Autodesk Inventor part; units mm, degrees
ref_plane "Work Plane5" through (-4.7625, 0, 3.175) normal (0, 0, 1) x (1, 0, 0)
ref_plane "YZ Plane" through (0, 0, 0) normal (1, 0, 0) x (0, 1, 0)
ref_plane "XZ Plane" through (0, 0, 0) normal (0, 1, 0) x (-1, 0, 0)
sketch "Sketch1" plane through (0, 0, 0) normal (0, 1, 0) x (-1, 0, 0)
  line L0 (-6.35, 12.7) -> (6.35, 12.7)
  line L1 (6.35, 12.7) -> (6.35, -12.7)
  line L2 (6.35, -12.7) -> (-6.35, -12.7)
  line L3 (-6.35, -12.7) -> (-6.35, 12.7)
  line L4 (-6.35, 12.7) -> (6.35, -12.7) construction
  line L5 (6.35, 12.7) -> (-6.35, -12.7) construction
  line L6 (-9.525, 19.05) -> (9.525, 19.05)
  line L7 (9.525, 19.05) -> (9.525, -19.05)
  line L8 (9.525, -19.05) -> (-9.525, -19.05)
  line L9 (-9.525, -19.05) -> (-9.525, 19.05)
  line L10 (-9.525, 19.05) -> (9.525, -19.05) construction
  line L11 (9.525, 19.05) -> (-9.525, -19.05) construction
  line L12 (6.35, 12.7) -> (6.35, 15.875)
  line L13 (6.35, 15.875) -> (9.525, 15.875)
  point P0 (0, 0)
  dimension "d0" = 12.7
  dimension "d1" = 25.4
extrude "Extrusion1" add sketch "Sketch1" along normal blind 3.175
sketch "Sketch2" plane through (0, 3.175, 0) normal (0, 1, 0) x (1, 0, 0)
  circle A0 centre (3.175, -9.525) radius 1.5875
  circle A1 centre (-3.175, 0) radius 1.5875
  circle A2 centre (0, 8.5298) radius 1.5
  line L0 (-4.318, -7.9375) -> (-2.032, -7.9375)
  line L1 (-2.032, -7.9375) -> (-2.032, -11.1125)
  line L2 (-2.032, -11.1125) -> (-4.318, -11.1125)
  line L3 (-4.318, -11.1125) -> (-4.318, -7.9375)
  line L4 (-4.318, -7.9375) -> (-2.032, -11.1125) construction
  line L5 (-2.032, -7.9375) -> (-4.318, -11.1125) construction
  line L6 (-9.525, 19.05) -> (-9.525, -19.05)
  line L7 (9.525, -19.05) -> (-9.525, -19.05)
  line L8 (-9.525, -19.05) -> (-9.525, 19.05)
  line L9 (-9.525, 19.05) -> (9.525, 19.05)
  line L10 (9.525, 19.05) -> (9.525, -19.05)
  line L11 (9.525, -19.05) -> (-9.525, 19.05) construction
  line L12 (-9.525, -19.05) -> (9.525, 19.05) construction
  point P0 (0, 0)
  point P1 (0, 0)
  dimension "d4" = 3.175
  dimension "d5" = 3.175
  dimension "d6" = 3
  dimension "d8" = 3.175
extrude "Extrusion2" add sketch "Sketch2" along normal blind 3.175
sketch "Sketch3" plane through (0, 6.35, 0) normal (0, 1, 0) x (1, 0, 0)
  line L0 (-9.525, 19.05) -> (-9.525, -19.05)
  line L1 (9.525, -19.05) -> (-9.525, -19.05)
  line L2 (-9.525, -19.05) -> (-9.525, 19.05)
  line L3 (-9.525, 19.05) -> (9.525, 19.05)
  line L4 (9.525, 19.05) -> (9.525, -19.05)
  line L5 (9.525, -19.05) -> (-9.525, 19.05) construction
  line L6 (-9.525, -19.05) -> (9.525, 19.05) construction
  line L7 (6.35, -12.7) -> (-6.35, -12.7)
  line L8 (-6.35, -12.7) -> (-6.35, 12.7)
  line L9 (-6.35, 12.7) -> (6.35, 12.7)
  line L10 (6.35, 12.7) -> (6.35, -12.7)
  line L11 (6.35, -12.7) -> (-6.35, 12.7) construction
  line L12 (-6.35, -12.7) -> (6.35, 12.7) construction
  point P0 (0, 0)
extrude "Extrusion3" add sketch "Sketch3" along normal blind 3.175
sketch "Sketch4" plane through (9.525, 0, -19.05) normal (0, 0, -1) x (-1, 0, 0)
  line L0 (12.7, 0) -> (6.35, 0)
  line L1 (6.35, 0) -> (6.35, 9.525)
  line L2 (6.35, 9.525) -> (12.7, 9.525)
  line L3 (12.7, 9.525) -> (12.7, 0)
  line L4 (12.7, 0) -> (6.35, 9.525) construction
  line L5 (6.35, 0) -> (12.7, 9.525) construction
  point P0 (9.525, 0)
  point P1 (9.525, 4.7625)
extrude "Extrusion4" add sketch "Sketch4" along normal blind 3.175
sketch "Sketch5" plane through (9.525, 0, -22.225) normal (0, 0, -1) x (-1, 0, 0)
  line L0 (4.7625, 0) -> (14.2875, 0)
  line L1 (14.2875, 0) -> (14.2875, 9.525)
  line L2 (14.2875, 9.525) -> (4.7625, 9.525)
  line L3 (4.7625, 9.525) -> (4.7625, 0)
  line L4 (4.7625, 0) -> (14.2875, 9.525) construction
  line L5 (14.2875, 0) -> (4.7625, 9.525) construction
  point P0 (9.525, 0)
  point P1 (9.525, 4.7625)
extrude "Extrusion5" add sketch "Sketch5" along normal blind 3.175
sketch "Sketch6" plane through (0, 9.525, 0) normal (0, 1, 0) x (1, 0, 0)
  line L0 (9.525, -19.05) -> (-9.525, -19.05)
  line L1 (-9.525, -19.05) -> (-9.525, -25.4)
  line L2 (9.525, -25.4) -> (9.525, -19.05)
  line L3 (3.175, -22.225) -> (4.7625, -22.225)
  line L4 (-4.7625, 25.4) -> (4.7625, 25.4)
  line L5 (4.7625, 22.225) -> (4.7625, 25.4)
  line L6 (-4.7625, -22.225) -> (-3.175, -22.225)
  line L7 (-3.175, -22.225) -> (-3.175, -25.4)
  line L8 (-4.7625, -22.225) -> (-4.7625, -19.05)
  line L9 (4.7625, -22.225) -> (4.7625, -19.05)
  line L10 (3.175, -22.225) -> (3.175, -25.4)
  line L11 (-9.525, -25.4) -> (-3.175, -25.4)
  line L12 (3.175, -25.4) -> (9.525, -25.4)
  point P0 (0, 0)
extrude "Extrusion6" add sketch "Sketch6" against normal blind 9.525
sketch "Sketch7" plane through (3.175, 9.525, 25.4) normal (0, 0, 1) x (1, 0, 0)
  circle A0 centre (9.35, -4.7625) radius 1.5
  line L0 (12.85, -5.0165) -> (12.85, -4.5085)
  line L1 (12.85, -4.5085) -> (12.85, 0) construction
  line L2 (12.85, 0) -> (6.35, 0) construction
  spline S0 degree 2 poles (12.85, -4.5085) (12.85, 0) (6.35, 0) knots 1 1 1 2 2 2
  line L3 (12.85, -5.0165) -> (12.85, -9.525) construction
  line L4 (12.85, -9.525) -> (6.35, -9.525) construction
  spline S1 degree 2 poles (12.85, -5.0165) (12.85, -9.525) (6.35, -9.525) knots 1 1 1 2 2 2
  line L5 (-3.175, -9.525) -> (-3.175, 0)
  line L6 (-7.9375, 0) -> (1.5875, 0)
  line L7 (6.35, 0) -> (6.35, -9.525)
  line L8 (6.35, -9.525) -> (6.35, 0)
  circle A1 centre (-15.7, -4.7625) radius 1.5
  line L9 (-19.2, -5.0165) -> (-19.2, -4.5085)
  line L10 (-19.2, -4.5085) -> (-19.2, 0) construction
  line L11 (-19.2, 0) -> (-12.7, 0) construction
  spline S2 degree 2 poles (-19.2, -4.5085) (-19.2, 0) (-12.7, 0) knots 1 1 1 2 2 2
  line L12 (-19.2, -5.0165) -> (-19.2, -9.525) construction
  line L13 (-19.2, -9.525) -> (-12.7, -9.525) construction
  spline S3 degree 2 poles (-19.2, -5.0165) (-19.2, -9.525) (-12.7, -9.525) knots 1 1 1 2 2 2
  line L14 (-12.7, 0) -> (-12.7, -9.525)
  line L15 (-12.7, -9.525) -> (-12.7, 0)
  point P0 (10.85, -4.7625)
  point P1 (-17.2, -4.7625)
  dimension "d25" = 3
extrude "Extrusion7" add sketch "Sketch7" against normal blind 3.175
ref_plane "Work Plane5" through (-4.7625, 0, 3.175) normal (0, 0, 1) x (1, 0, 0)
mirror "Mirror1" about plane through (-4.7625, 0, 3.175) normal (0, 0, 1) of "Extrusion7"
properties part number "SlottedCarrierFull"
Input: part model. Units: mm. Frame: model coordinates. A direction names the side the tool comes from. Coordinates: 2 decimals unless noted, no trailing zeros. Loops run counter-clockwise (first coordinate to the right, second up) from the corner with the lowest first, then second, coordinate; pieces in that order, holes last.
Q1. Section B-B, the plane x = 0. Return the cut outline in (y, z) (3 decimals), and give its area (3 significant figures).
Results are:
outline: (0, -25.4) - (9.525, -25.4) - (9.525, -12.7) - (6.35, -12.7) - (6.35, -10.03) - (3.175, -10.03) - (3.175, -12.7) - (0, -12.7) - close; (0, 12.7) - (3.175, 12.7) - (3.175, -7.03) - (6.35, -7.03) - (6.35, 12.7) - (9.525, 12.7) - (9.525, 19.05) - (0, 19.05) - close
area: 253 mm2
Q2. Line query: line 1 along X through (y, z) = (6.75, -5) (3 decimals); line 2 along Z through (x, y) = (5, 1); line 3 along Z through (x, y) = (-13, 6.5) (3 decimals). Output: solid intervals per line, ascending.
Results are:
line 1: x = -9.525 to -6.35, 6.35 to 9.525
line 2: z = -19.05 to -12.7, 12.7 to 25.4
line 3: z = -19.05 to -15.875, 22.225 to 25.4
Q3. Mould query, pull axis X, two halves, no side actions, for faces 4 (the flat face through (9.525, 5, 3)), 5 (the cylindrical face through (11.026, 4.697, -17.485)), 6 (the flat face through (4, 5, -22.225)), 7 (the flat face through (-4.762, 5, -24)). Classes: +X half, -X half, draft (parallel to the pull), parting line (faces both ways), or undercut.
Results are:
face 4: +X half
face 5: undercut
face 6: draft
face 7: -X half
Q4. Contact query for flat-ended pins moving along their axis: pin 1 (5 mm diameter, centred on x = 9.5, y = 5, fed in from -Z); pin 2 (4 mm diameter, centred on y = 4.5, z = -10.5, fed in from -X) (3 decimals); pin 3 (2 mm diameter, centred on y = 2, z = -3.5, fed in from +X) (3 decimals). Output: stop coordinate, or through.
Results are:
pin 1: stops at z = -19.05
pin 2: stops at x = -9.525
pin 3: stops at x = 9.525
Q5. Section D-D, the plane x = -8. Return the cut outline in (y, z) (3 decimals).
Results are:
outline: (0, -19.05) - (9.525, -19.05) - (9.525, 25.4) - (0, 25.4) - close
Q6. Set-up query: faces 1 (the flat face through (0, 6.35, 0)), 2 (the flat face through (10, 5, -19.05)), 3 (the flat face through (4, 5, 22.225)). Return all of +Z, -Z, +X, -X, +Y, -Y with unobstructed straight access to the full face (end or side cutting, diameter ignored); none if empty.
Results are:
face 1: +Y
face 2: +X, +Y, -Y
face 3: +Y, -Y
Q7. Section C-C, the plane y = 3.75. Give the number of separate pieces and of enclosed holes in the cut face, and give its area (3 significant figures).
Results are:
separate pieces: 5
enclosed holes: 4
area: 870 mm2
